Autodesk Inventor part; units mm, degrees
ref_plane "YZ Plane" through (0, 0, 0) normal (1, 0, 0) x (0, 1, 0)
ref_plane "XZ Plane" through (0, 0, 0) normal (0, 1, 0) x (-1, 0, 0)
ref_plane "XY Plane" through (0, 0, 0) normal (0, 0, 1) x (1, 0, 0)
sketch "Sketch1" plane through (0, 0, 0) normal (1, 0, 0) x (0, 1, 0)
  line L0 (174.9139, 1066.8) -> (200.3139, 1066.8)
  line L1 (200.3139, 1066.8) -> (200.3139, 812.8)
  line L2 (200.3139, 812.8) -> (403.5139, 304.8)
  line L3 (403.5139, 304.8) -> (403.5139, -304.8)
  line L4 (403.5139, -304.8) -> (200.3139, -812.8)
  line L5 (200.3139, -812.8) -> (200.3139, -1066.8)
  line L6 (174.9139, 1066.8) -> (174.9139, 812.8)
  line L7 (174.9139, 812.8) -> (378.1139, 304.8)
  line L8 (378.1139, 304.8) -> (378.1139, -304.8)
  line L9 (174.9139, -935.25) -> (174.9139, 993.0491) construction
  line L10 (174.9139, 681.698) -> (174.9139, -514.0179) construction
  line L11 (200.3139, -1066.8) -> (174.9139, -1066.8)
  line L12 (378.1139, -304.8) -> (174.9139, -812.8)
  line L13 (174.9139, -812.8) -> (174.9139, -1066.8)
  point P0 (0, 0)
  dimension "d0" = 254
  dimension "d1" = 508
  dimension "d2" = 609.6
  dimension "d3" = 508
  dimension "d4" = 254
  dimension "d6" = 304.8
  dimension "d8" = 25.4
  dimension "d10" = 203.2
  dimension "d26" = 25.4
extrude "Extrusion1" add sketch "Sketch1" along normal mid plane 609.6
sketch "Sketch2" plane through (-304.8, 200.3139, -812.8) normal (0, 1, 0) x (1, 0, 0)
  circle A0 centre (304.8, 139.7) radius 95.25
  line L0 (609.6, 254) -> (0, 254)
  line L1 (0, 0) -> (0, 254)
  circle A1 centre (304.8, -1765.3) radius 95.25
  line L2 (609.6, -1879.6) -> (0, -1879.6)
  line L3 (609.6, -1625.6) -> (609.6, -1879.6)
  point P0 (304.8, -812.8)
  dimension "d13" = 190.5
  dimension "d14" = 114.3
  dimension "d15" = 304.8
  dimension "d16" = 190.5
  dimension "d17" = 114.3
  dimension "d18" = 304.8
extrude "Extrusion2" cut sketch "Sketch2" against normal up to next
sketch "Sketch3" plane through (-304.8, 403.5139, 304.8) normal (0, 1, 0) x (1, 0, 0)
  circle A0 centre (304.8, 304.8) radius 146.05
  line L0 (0, 609.6) -> (0, 0)
  line L1 (609.6, 609.6) -> (0, 609.6)
  point P0 (304.8, 304.8)
  dimension "d21" = 292.1
  dimension "d22" = 304.8
  dimension "d23" = 304.8
extrude "Extrusion3" cut sketch "Sketch3" against normal up to next
properties part number "Up_cam_support"
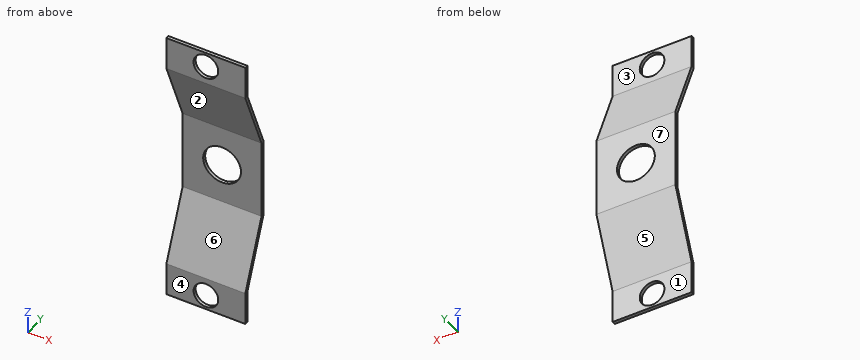
The model under review builds one solid part; all positions refer to its coordinate system, in mm. Face numbers are marked on the shaded views. A direction names the side the tool comes from. Round coordinates to 2 decimals unless told otherwise and drop trailing zeros. Loops run counter-clockwise (first coordinate to the right, second up) from the corner with the lowest first, then second, coordinate; pieces in that order, holes last. Notation, with made-up numbers: (79.5, 78) - (92.5, 78) arc R18 cw to (92.5, 89) - close; hole circle Ø4 at (-2.75, 45). An arc over 180 degrees is marked (long way). Write each question's results on one line, items separated by ' | '. Start each with the question number.
Q1. Draft analysis for pull direction Z (two halves, no side actions). For the marked faces 5, 6 and 7, state which applies: pulls with the +Z half, pulls with the -Z half, needs draft (parallel to the pull), parting line crosses it, or undercut.
Q2. Take a section at D-D on x = -266. Give the boundary of the cut face in (y, z), plus the area to 3 significant figures.
Q3. Take a section at A-A on z = 952.5. Give the boundary of the cut face in (x, y), plus the area to 3 significant figures.
Q4. Take a section at B-B on x = 0. Give the boundary of the cut face in (y, z), plus the area to 3 significant figures.
Q5. Insertion check: P1, Ø10, axis at x = -71, z = -371, coming from the +Y side; P2, Ø2, axis at x = -28.5, z = -207, coming from the -Y side. Each pin has a flat end and moves straight along its axis. Give the tip position at first contact, or say it passes through.
Q6. Tool access review of the marked faces 1, 2, 3 and 4: name each direction out of +Z, -Z, +X, -X, +Y, -Y from which nothing blocks a thin tool from reaching the whole face with its end or side.
Q7. Wall thickness on line 1 along X through (y, z) = (393.75, 0); line 2 along X through (y, z) = (190, 952); line 3 along Z through (x, y) = (193.5, 346): over which ranges is each line inside the solid? List them lowest first. Write a range as [from, to].
Q8. Take a section at C-C on y = 256.5. Give the boundary of the cut face in (x, z).
Data:
1) face 5: pulls with the -Z half | face 6: undercut | face 7: needs draft
2) outline: (174.91, -1066.8) - (200.31, -1066.8) - (200.31, -812.8) - (403.51, -304.8) - (403.51, 304.8) - (200.31, 812.8) - (200.31, 1066.8) - (174.91, 1066.8) - (174.91, 812.8) - (378.11, 304.8) - (378.11, -304.8) - (174.91, -812.8) - close | area: 54,200 mm²
3) outline: (-304.8, 174.91) - (-95.25, 174.91) - (-95.25, 200.31) - (-304.8, 200.31) - close; (95.25, 174.91) - (304.8, 174.91) - (304.8, 200.31) - (95.25, 200.31) - close | area: 10,600 mm²
4) outline: (174.91, -1066.8) - (200.31, -1066.8) - (200.31, -1047.75) - (174.91, -1047.75) - close; (174.91, -857.25) - (200.31, -857.25) - (200.31, -812.8) - (403.51, -304.8) - (403.51, -146.05) - (378.11, -146.05) - (378.11, -304.8) - (174.91, -812.8) - close; (174.91, 812.8) - (378.11, 304.8) - (378.11, 146.05) - (403.51, 146.05) - (403.51, 304.8) - (200.31, 812.8) - (200.31, 857.25) - (174.91, 857.25) - close; (174.91, 1047.75) - (200.31, 1047.75) - (200.31, 1066.8) - (174.91, 1066.8) - close | area: 37,100 mm²
5) P1: stops at y = 379.03 | P2: stops at y = 378.11
6) face 1: -Z, +X, -X, +Y | face 2: +X, -X, -Y | face 3: +Z, +X, -X, +Y | face 4: +Z, -Z, +X, -X, -Y
7) line 1: x = [-304.8, -146.05], [146.05, 304.8] | line 2: x = [-304.8, -95.25], [95.25, 304.8] | line 3: z = [-448.58, -385.08], [385.08, 448.58]
8) outline: (-304.8, -672.33) - (304.8, -672.33) - (304.8, -608.83) - (-304.8, -608.83) - close; (-304.8, 608.83) - (304.8, 608.83) - (304.8, 672.33) - (-304.8, 672.33) - close
